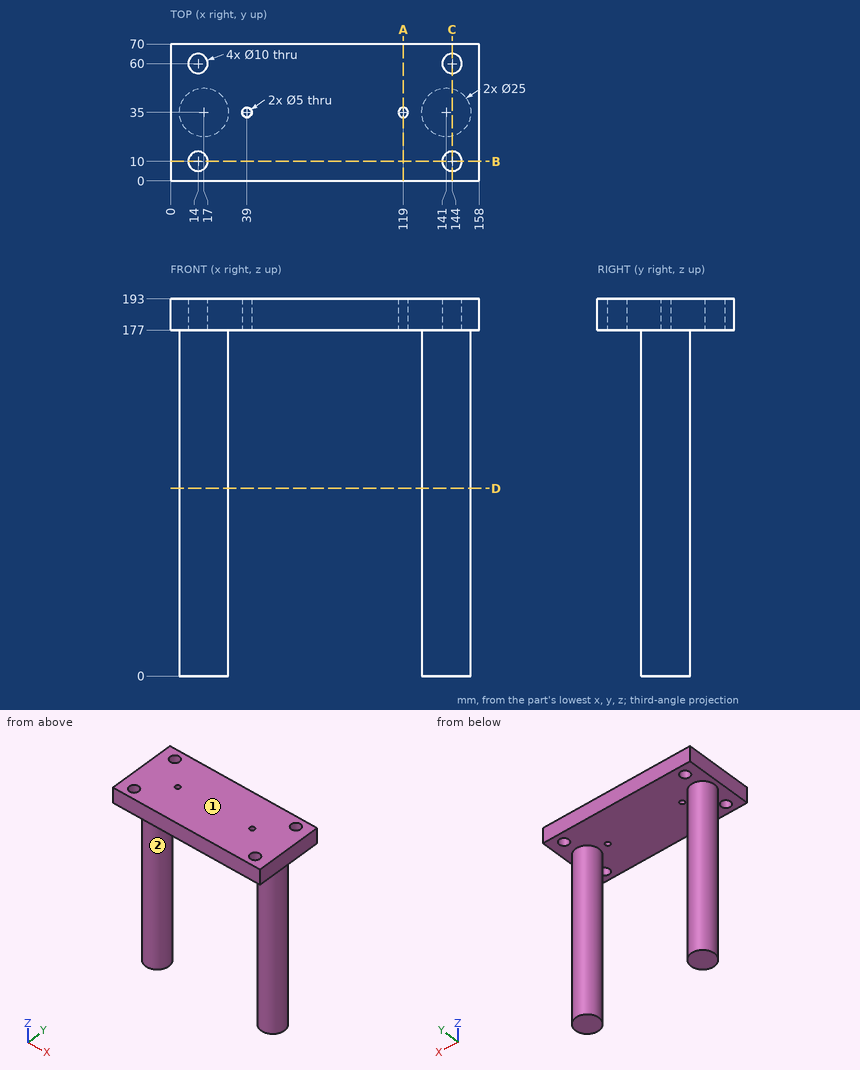
Source: three-view drawing plus pictorial views. Frame: mm from the lowest corner of the part. A direction names the side the tool comes from. Coordinates: 2 decimals unless noted, no trailing zeros. Write each loop counter-clockwise with the first axis right and the second up, starting at its lowest first coordinate (ties: lowest second). Pieces come first, ordered by that corner, then holes. Notation, with made-up numbers: (15, 12) -> (59, 12) arc R11 ccw to (59, 19) -> close; hole circle Ø7 at (2.25, 61.5). An arc over 180 degrees is marked (long way). Answer as a JSON object with one key per item and string values.
1. First-contact query: P1, Ø4.5, axis at x = 119, y = 35, coming from the +Z side; P2, Ø6, axis at x = 22.5, z = 153.5, coming from the +Y side; P3, Ø4, axis at y = 30, z = 32, coming from the +X side; P4, Ø12, axis at x = 129, y = 57, coming from the -Z side. Flat tips, straight axial feed; report the tip coordinate or a pass-through.
Result set:
{"P1": "passes through", "P2": "stops at y = 47.25", "P3": "stops at x = 153.13", "P4": "stops at z = 177"}
2. Material intervals for line 1 (Y direction, x = 144, z = 182); line 2 (Y direction, x = 119, z = 187); line 3 (Z direction, x = 53, y = 27), sorted ascending. Write a range as from..to.
Result set:
{"line 1": "y = 0..5, 15..55, 65..70", "line 2": "y = 0..32.5, 37.5..70", "line 3": "z = 177..193"}
3. Access query for the marked faces 1 and 2. Directions: +Z, -Z, +X, -X, +Y, -Y. A direction counts if a zero-diameter tool reaches every point of the face in a straight line with its end or side. Return the directions, or none.
Result set:
{"face 1": "+Z, +X, -X, +Y, -Y", "face 2": "-Z"}
4. Section A-A on x = 119. Return the cut outline in (y, z).
Result set:
{"outline": "(0, 177) -> (32.5, 177) -> (32.5, 193) -> (0, 193) -> close; (37.5, 177) -> (70, 177) -> (70, 193) -> (37.5, 193) -> close"}
5. Section C-C on x = 144. Return the cut outline in (y, z), then the cut area to 3 significant figures.
Result set:
{"outline": "(0, 177) -> (5, 177) -> (5, 193) -> (0, 193) -> close; (15, 177) -> (22.87, 177) -> (22.87, 0) -> (47.13, 0) -> (47.13, 177) -> (55, 177) -> (55, 193) -> (15, 193) -> close; (65, 177) -> (70, 177) -> (70, 193) -> (65, 193) -> close", "area": "5,100 mm2"}
6. Section B-B on y = 10. Return the cut outline in (x, z).
Result set:
{"outline": "(0, 177) -> (9, 177) -> (9, 193) -> (0, 193) -> close; (19, 177) -> (139, 177) -> (139, 193) -> (19, 193) -> close; (149, 177) -> (158, 177) -> (158, 193) -> (149, 193) -> close"}
7. Section D-D on z = 96. Return the cut outline in (x, y).
Result set:
{"outline": "circle Ø25 at (17, 35); circle Ø25 at (141, 35)"}
